from build123d import *

# Parameters (mm, degrees)
ESQUISSE1_R                  = 11.1
ESQUISSE1_R_2                = 1.65
ESQUISSE1_W                  = 8.6
ESQUISSE1_H                  = 4.6
ESQUISSE1_W_2                = 4.6
ESQUISSE1_H_2                = 8.6
BOSS_EXTRU_1_DEPTH           = 13
CHANFREIN1_SIZE              = 2
ESQUISSE6_R                  = 2.6
ENL_V_MAT_EXTRU_4_DEPTH      = 17
R_P_TITION_CIRCULAIRE1_COUNT = 4
ESQUISSE7_R                  = 2.5
BOSS_EXTRU_2_DEPTH           = 10
CONG_1_R                     = 2


with BuildPart() as part:
    # Esquisse1 → Boss.-Extru.1 (new body)
    with BuildSketch(Plane.XY):
        with BuildLine():
            Line((-6.105930323, 29.167749568), (-6.105930323, 23.762922109))
            Line((-6.105930323, 23.762922109), (6.105930323, 23.762922109))
            Line((6.105930323, 23.762922109), (6.105930323, 29.167749568))
            ThreePointArc((6.105930323, 29.167749568), (21.071782079, 21.071782079), (29.167749568, 6.105930323))
            Line((29.167749568, 6.105930323), (23.762922109, 6.105930323))
            Line((23.762922109, 6.105930323), (23.762922109, -6.105930323))
            Line((23.762922109, -6.105930323), (29.167749568, -6.105930323))
            ThreePointArc((29.167749568, -6.105930323), (21.071782079, -21.071782079), (6.105930323, -29.167749568))
            Line((6.105930323, -29.167749568), (6.105930323, -23.762922109))
            Line((6.105930323, -23.762922109), (-6.105930323, -23.762922109))
            Line((-6.105930323, -23.762922109), (-6.105930323, -29.167749568))
            ThreePointArc((-6.105930323, -29.167749568), (-21.071782079, -21.071782079), (-29.167749568, -6.105930323))
            Line((-29.167749568, -6.105930323), (-23.762922109, -6.105930323))
            Line((-23.762922109, -6.105930323), (-23.762922109, 6.105930323))
            Line((-23.762922109, 6.105930323), (-29.167749568, 6.105930323))
            ThreePointArc((-29.167749568, 6.105930323), (-21.071782079, 21.071782079), (-6.105930323, 29.167749568))
        make_face()
        with Locations(Location((0, 0, 0), (0, 0, 180))):
            Circle(ESQUISSE1_R, mode=Mode.SUBTRACT)
        with Locations(Location((-10.960155108, 18.983545507, 0), (0, 0, 180))):
            Circle(ESQUISSE1_R_2, mode=Mode.SUBTRACT)
        with Locations(Location((18.983545507, 10.960155108, 0), (0, 0, 180))):
            Circle(ESQUISSE1_R_2, mode=Mode.SUBTRACT)
        with Locations(Location((10.960155108, -18.983545507, 0), (0, 0, 180))):
            Circle(ESQUISSE1_R_2, mode=Mode.SUBTRACT)
        with Locations(Location((-18.983545507, -10.960155108, 0), (0, 0, 180))):
            Circle(ESQUISSE1_R_2, mode=Mode.SUBTRACT)
        with Locations((0, 16.762922109)):
            Rectangle(ESQUISSE1_W, ESQUISSE1_H, mode=Mode.SUBTRACT)
        with Locations((16.762922109, 0)):
            Rectangle(ESQUISSE1_W_2, ESQUISSE1_H_2, mode=Mode.SUBTRACT)
        with Locations((0, -16.762922109)):
            Rectangle(ESQUISSE1_W, ESQUISSE1_H, mode=Mode.SUBTRACT)
        with Locations((-16.762922109, 0)):
            Rectangle(ESQUISSE1_W_2, ESQUISSE1_H_2, mode=Mode.SUBTRACT)
    extrude(amount=BOSS_EXTRU_1_DEPTH)

    # Chanfrein1
    chanfrein1_edges = [part.edges().sort_by_distance(p)[0] for p in [
        (-9.310155108, 18.983545507, 13),
        (20.633545507, 10.960155108, 13),
        (12.610155108, -18.983545507, 13),
        (-17.333545507, -10.960155108, 13),
    ]]
    chamfer(chanfrein1_edges, length=CHANFREIN1_SIZE)

    # Esquisse6 → Enlèv. mat.-Extru.4 (cut)
    with BuildSketch(Plane.ZY.offset(23.762922109)):
        with Locations((7, 0)):
            Circle(ESQUISSE6_R)
    enl_v_mat_extru_4 = extrude(amount=-ENL_V_MAT_EXTRU_4_DEPTH, mode=Mode.SUBTRACT)

    # Répétition circulaire1: Enlèv. mat.-Extru.4 ×4 about axis
    r_p_tition_circulaire1_axis = Axis((0, 0, 0), (0, 0, -1))
    for i in range(1, R_P_TITION_CIRCULAIRE1_COUNT):
        add(enl_v_mat_extru_4.rotate(r_p_tition_circulaire1_axis, i * 360 / R_P_TITION_CIRCULAIRE1_COUNT), mode=Mode.SUBTRACT)

    # Esquisse7 → Boss.-Extru.2 (add)
    with BuildSketch(Plane.XY.offset(13)):
        with Locations((-13.925584753, 9.750799418)):
            Circle(ESQUISSE7_R)
        with Locations((9.750799418, 13.925584753)):
            Circle(ESQUISSE7_R)
        with Locations((13.925584753, -9.750799418)):
            Circle(ESQUISSE7_R)
        with Locations((-9.750799418, -13.925584753)):
            Circle(ESQUISSE7_R)
    extrude(amount=BOSS_EXTRU_2_DEPTH)

    # Congé1
    cong_1_edges = [part.edges().sort_by_distance(p)[0] for p in [
        (-16.425584753, 9.750799418, 13),
        (7.250799418, 13.925584753, 13),
        (11.425584753, -9.750799418, 13),
        (-12.250799418, -13.925584753, 13),
    ]]
    fillet(cong_1_edges, radius=CONG_1_R)


solid = part.part
Can you work these out from the model? Positions are in its coordinate system, mm. A direction names the side the tool comes from. Round coordinates to 2 decimals unless told otherwise and drop trailing zeros. Order: outer loops, then holes, each group sorted by start corner. A loop starts at its lowest first (then second) coordinate and runs counter-clockwise, first axis right, second up. Notation, with made-up numbers: (80.25, 30) -> (118.25, 30) arc R34 cw to (118.25, 61) -> close; hole circle Ø1 at (78, 38). An arc over 180 degrees is marked (long way). Write each question's results on one line, items separated by ' | '. Start each with the question number.
Item 1: Which directions (+Z, -Z, +X, -X, +Y, -Y) give clear straight access to the entire face, cutting with the end or side of a thin tool? Please do faces 1 (the flat face through (-23.763, 3, 6)), 2 (the flat face through (2, 14.463, 5)), 3 (the flat face through (3, 23.763, 6)).
Item 2: Thinking about a two-plate mould opening in Y: for faces 4 (the cylindrical face through (-0.1, -12.7, 4.4)), 5 (the cylindrical face through (-21.24, 20.9, 6.41)), 6 (the cylindrical face through (12.7, -0.1, 4.4)), which applies, +Y half, -Y half, draft (parallel to the pull), parting line (faces both ways), or undercut?
Item 3: If we section it at A-A, the plane x = 0: State how many separate pieces and enclosed holes the cut face has, then the cut area to 3 significant figures.
Item 4: If we section it at C-C, the plane x = -26: Write out the boundary of the cut face in (y, z), then the cut area to 3 significant figures.
Item 5: Please list where these lines run through material, in increasing order: L1, parallel to X at y = 11.95, z = 7; L2, parallel to X at y = 2.5, z = 4.75; L3, parallel to Y at x = -18, z = 8.25.
Item 6: Will these pins go through, and if not, where does the flat tip stop? pin 1 (7 mm diameter, centred on x = 0.5, z = 7.5, fed in from +Y); pin 2 (2.5 mm diameter, centred on x = 26.5, z = 4.5, fed in from -Y); pin 3 (9.5 mm diameter, centred on y = 0, z = 7, fed in from +X).
Results:
1) face 1: +Z, -Z, -X | face 2: +Z, -Z | face 3: +Z, -Z, +Y
2) face 4: draft | face 5: +Y half | face 6: undercut
3) separate pieces: 8 | enclosed holes: 0 | area: 126 mm2
4) outline: (-14.56, 0) -> (-6.11, 0) -> (-6.11, 13) -> (-14.56, 13) -> close; (6.11, 0) -> (14.56, 0) -> (14.56, 13) -> (6.11, 13) -> close | area: 220 mm2
5) L1: x = -27.3 to -2.6, 2.6 to 17.66, 20.3 to 27.3 | L2: x = -23.76 to -19.06, -14.46 to -10.81, 10.81 to 14.46, 19.06 to 23.76 | L3: y = -23.75 to -12.28, -9.64 to -4.3, 4.3 to 23.75
6) pin 1: stops at y = 23.76 | pin 2: stops at y = -15.83 | pin 3: stops at x = 23.76
